from build123d import *

# Parameters (mm, degrees)
PAD_DEPTH       = 170
SKETCH001_W     = 16
SKETCH001_H     = 16
POCKET_DEPTH    = 20
POCKET001_DEPTH = 20
SKETCH005_R     = 3.7
POCKET002_DEPTH = 2
SKETCH006_R     = 2.4
POCKET003_DEPTH = 4
SKETCH007_W     = 5
SKETCH007_H     = 130
PAD001_DEPTH    = 2


with BuildPart() as part:
    # Sketch → Pad (new body)
    with BuildSketch(Plane.XY):
        Polygon((0, 20), (0, 0), (20, 0), (20, 4), (4, 20), align=None)
    extrude(amount=PAD_DEPTH)

    # Sketch001 (on Face7 of Pad) → Pocket (cut)
    with BuildSketch(Plane.XY.offset(170)):
        with Locations((12, 12)):
            Rectangle(SKETCH001_W, SKETCH001_H)
    extrude(amount=-POCKET_DEPTH, mode=Mode.SUBTRACT)

    # Sketch004 → Pocket001 (cut)
    with BuildSketch(Plane(origin=(0, 0, 0), x_dir=(1, 0, 0), z_dir=(0, 0, -1))):
        Polygon((4, -4), (4, -20), (20, -4), align=None)
    extrude(amount=-POCKET001_DEPTH, mode=Mode.SUBTRACT)

    # Sketch005 → Pocket002 (cut)
    with BuildSketch(Plane.YZ.offset(4)):
        with Locations((12, 160)):
            Circle(SKETCH005_R)
        with Locations((12, 10)):
            Circle(SKETCH005_R)
    extrude(amount=-POCKET002_DEPTH, mode=Mode.SUBTRACT)

    # Sketch006 → Pocket003 (cut)
    with BuildSketch(Plane.YZ.offset(4)):
        with Locations((12, 10)):
            Circle(SKETCH006_R)
        with Locations((12, 160)):
            Circle(SKETCH006_R)
    extrude(amount=-POCKET003_DEPTH, mode=Mode.SUBTRACT)

    # Sketch007 → Pad001 (join)
    with BuildSketch(Plane(origin=(12, 12, 0), x_dir=(-0.707107, 0.707107, 0), z_dir=(0.707107, 0.707107, 0))):
        with Locations((-8.813708, 85)):
            Rectangle(SKETCH007_W, SKETCH007_H)
        with Locations((8.813708, 85)):
            Rectangle(SKETCH007_W, SKETCH007_H)
    extrude(amount=PAD001_DEPTH)


solid = part.part
Could you check a few things on this model? Use its own coordinates, in mm. A direction names the side the tool comes from. Give positions to 0.01 mm unless a question says otherwise; leave off trailing zeros. Write each loop counter-clockwise with the first axis right and the second up, starting at its lowest first coordinate (ties: lowest second). Pieces come first, ordered by that corner, then holes. Notation, with made-up numbers: (56, 18.5) - (64, 18.5) arc R33 ccw to (64, 51.5) - close; hole circle Ø8 at (9.25, 73). An arc over 180 degrees is marked (long way). Use CSV: the item, a comma, the result in double quotes. Start each with the question number.
Item 1: For faces 4 (the face through (2, 11.1, 157.6)), 5 (the face through (4, 8, 12)), 6 (the face through (20, 2, 84)), which set-ups out of +Z, -Z, +X, -X, +Y, -Y let a thin tool reach every point of the face, with its end or its side?
Item 2: If we mould it in two halves opening along Y, with no side actions, what happens to faces 1 (the face through (1.01, 11.69, 162.38)), 2 (the face through (2, 20, 84)), 3 (the face through (5, 3, 0))? For each: pulls with the +Y half, pulls with the -Y half, needs draft (parallel to the pull), parting line crosses it, or undercut.
Item 3: I want a section at C-C, the plane x = 11.25. Please give me the cut outline in (y, z), then the cut area to 3 significant figures.
Item 4: I want a section at A-A, the plane y = 12. Please give me the cut outline in (x, z), then the cut area to 3 significant figures.
Item 5: I'm going to push flat-ended pins straight in: pin 1 (1.2 mm diameter, centred on x = 1.5, z = 62.5, fed in from +Y); pin 2 (5 mm diameter, centred on x = 16, y = 9, fed in from +Z); pin 3 (10 mm diameter, centred on y = 14, z = 132.5, fed in from +X); pin 4 (4.5 mm diameter, centred on y = 12, z = 160, fed in from +X). Where does each tip first touch, or does it pass through?
Item 6: I want a section at D-D, the plane z = 92. Please give me the cut outline in (x, y), then the cut area to 3 significant figures.
Item 7: If I drill on line 1 along Z through (x, y) = (1.45, 12); line 2 along Z through (x, y) = (2.9, 12); line 3 along Y through (x, z) = (1.25, 160), over which ranges is the centre line in solid material (lowest first)?
Item 8: I want a section at B-B, the plane z = 10. Please give me the cut outline in (x, y).
Findings:
1,face 4,"+X"
1,face 5,"-Z, +X, +Y"
1,face 6,"+Z, -Z, +X, -Y"
2,face 1,"undercut"
2,face 2,"pulls with the +Y half"
2,face 3,"needs draft"
3,outline,"(0, 0) - (4, 0) - (4, 20) - (12.75, 20) - (12.75, 150) - (4, 150) - (4, 170) - (0, 170) - close"
3,area,"1,820 mm2"
4,outline,"(0, 0) - (4, 0) - (4, 6.3) - (2, 6.3) - (2, 7.6) - (0, 7.6) - close; (0, 12.4) - (2, 12.4) - (2, 13.7) - (4, 13.7) - (4, 20) - (12, 20) - (12, 150) - (4, 150) - (4, 156.3) - (2, 156.3) - (2, 157.6) - (0, 157.6) - close; (0, 162.4) - (2, 162.4) - (2, 163.7) - (4, 163.7) - (4, 170) - (0, 170) - close"
4,area,"1,670 mm2"
5,pin 1,"stops at y = 20"
5,pin 2,"stops at z = 150"
5,pin 3,"stops at x = 15"
5,pin 4,"passes through"
6,outline,"(0, 0) - (20, 0) - (20, 4) - (21.41, 5.41) - (17.88, 8.95) - (16.46, 7.54) - (7.54, 16.46) - (8.95, 17.88) - (5.41, 21.41) - (4, 20) - (0, 20) - close"
6,area,"292 mm2"
7,line 1,"z = 0 to 7.6, 12.4 to 157.6, 162.4 to 170"
7,line 2,"z = 0 to 6.3, 13.7 to 156.3, 163.7 to 170"
7,line 3,"y = 0 to 9.6, 14.4 to 20"
8,outline,"(0, 0) - (20, 0) - (20, 4) - (4, 4) - (4, 8.3) - (2, 8.3) - (2, 9.6) - (0, 9.6) - close; (0, 14.4) - (2, 14.4) - (2, 15.7) - (4, 15.7) - (4, 20) - (0, 20) - close"
